Geometry check sheet. Reference: the model listing, model coordinates, mm. Face numbers are marked on the shaded views. A direction names the side the tool comes from. Round coordinates to 2 decimals unless told otherwise and drop trailing zeros. Order: outer loops, then holes, each group sorted by start corner. A loop starts at its lowest first (then second) coordinate and runs counter-clockwise, first axis right, second up.
(1) Sectioned sample at D-D (y = -21). Record the boundary of the cut face in (x, z).
(2) Sectioned sample at C-C (x = -4.5). Record the boundary of the cut face in (y, z), plus the area to 3 significant figures.
(3) Release check for a two-part mould opening along Z. For the marked faces 4, 5 and 6 record: +Z half, -Z half, draft (parallel to the pull), parting line (faces both ways), or undercut.
(4) Material ranges on line 1 along Y through (x, z) = (-3.75, -8); line 2 along Y through (x, z) = (6.25, -2); line 3 along Y through (x, z) = (2.25, -4), recorded low to high.
(5) Set-up check for the marked faces 1, 2 and 3: record each of +Z, -Z, +X, -X, +Y, -Y from which the full face is reachable in a straight line by a thin tool's end or side.
(6) Go/stop test with flat-tipped pins: pin 1 (2 mm diameter, centred on y = 9, z = 2, fed in from +X); pin 2 (1.5 mm diameter, centred on y = -34.5, z = 1, fed in from -X); pin 3 (4 mm diameter, centred on y = -15, z = -4.5, fed in from +X). Record where each tip stops, or that it passes through.
(7) Sectioned sample at A-A (y = -37). Record the boundary of the cut face in (x, z).
from build123d import *

# Parameters (mm, degrees)
CBORE_FOR_M3_SHCS1_D           = 3.4
CBORE_FOR_M3_SHCS1_DEPTH       = 8.5
CBORE_FOR_M3_SHCS1_CBORE_D     = 6.5
CBORE_FOR_M3_SHCS1_CBORE_DEPTH = 3
M3X0_5_TAPPED_HOLE1_D          = 2.5
CUT_EXTRUDE1_DEPTH             = 47.216880128
CUT_EXTRUDE1_DEPTH_BACK        = 47.216880128
SKETCH10_W                     = 1
SKETCH10_H                     = 15
CUT_EXTRUDE2_DEPTH             = 10


with BuildPart() as part:
    # Sketch1 → Revolve1 (revolve)
    with BuildSketch(Plane.XY):
        Polygon((-8.5, -44), (-8.5, -15.8), (-9.5, -15.8), (-9.5, -14), (-8.5, -14), (-8.5, 0), (-10, 0), (-10, 1.5), (-8.5, 1.5), (-8.5, 13.5), (-10, 13.5), (-10, 15), (0, 15), (0, -30), (-4, -30), (-4, -44), align=None)
    revolve(axis=Axis((0, 15, 0), (0, -1, 0)))

    # CBORE for M3 SHCS1
    with Locations(Plane.XY.offset(8.5)):
        with Locations((6.25, -37)):
            CounterBoreHole(CBORE_FOR_M3_SHCS1_D / 2, CBORE_FOR_M3_SHCS1_CBORE_D / 2, CBORE_FOR_M3_SHCS1_CBORE_DEPTH, depth=CBORE_FOR_M3_SHCS1_DEPTH)

    # M3x0.5 Tapped Hole1 (through all)
    with Locations(Plane.XY):
        with Locations((6.25, -37)):
            Hole(M3X0_5_TAPPED_HOLE1_D / 2)

    # Sketch10 → Cut-Extrude1 (cut, two sides: drawn at the far end of the back side and taken through both)
    with BuildSketch(Plane(origin=(0, 0, 0), x_dir=(0, 0, -1), z_dir=(1, 0, 0)).offset(-CUT_EXTRUDE1_DEPTH_BACK)):
        with Locations((0, -37.5)):
            Rectangle(SKETCH10_W, SKETCH10_H)
    extrude(amount=CUT_EXTRUDE1_DEPTH + CUT_EXTRUDE1_DEPTH_BACK, mode=Mode.SUBTRACT)

    # Sketch10<3> → Cut-Extrude2 (cut)
    with BuildSketch(Plane(origin=(0, 0, 0), x_dir=(0, 0, -1), z_dir=(1, 0, 0))):
        Polygon((-0.5, -30), (0.5, -30), (9.5, -30), (9.5, -29), (-9.5, -29), (-9.5, -30), align=None)
    extrude(amount=CUT_EXTRUDE2_DEPTH, mode=Mode.SUBTRACT)


solid = part.part
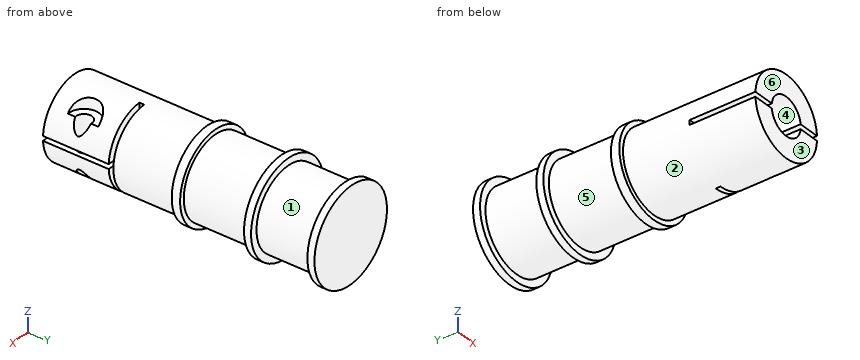
Answer below:
1. outline: circle Ø17 at (0, 0)
2. outline: (-44, -7.21) - (-15.8, -7.21) - (-15.8, -8.37) - (-14, -8.37) - (-14, -7.21) - (0, -7.21) - (0, -8.93) - (1.5, -8.93) - (1.5, -7.21) - (13.5, -7.21) - (13.5, -8.93) - (15, -8.93) - (15, 8.93) - (13.5, 8.93) - (13.5, 7.21) - (1.5, 7.21) - (1.5, 8.93) - (0, 8.93) - (0, 7.21) - (-14, 7.21) - (-14, 8.37) - (-15.8, 8.37) - (-15.8, 7.21) - (-44, 7.21) - (-44, 0.5) - (-30, 0.5) - (-30, -0.5) - (-44, -0.5) - close
2. area: 851 mm2
3. face 4: undercut
3. face 5: parting line
3. face 6: draft
4. line 1: y = -15.8 to -14, 0 to 1.5, 13.5 to 15
4. line 2: y = -44 to -38.25, -35.75 to -30, -29 to 15
4. line 3: y = -44 to -30, -29 to 15
5. face 1: none
5. face 2: -Y
5. face 3: +Z, -Z, +X, -X, -Y
6. pin 1: stops at x = 8.44
6. pin 2: stops at x = -8.49
6. pin 3: stops at x = 9.17
7. outline: (-8.49, -0.5) arc R8.5 ccw to (5, -6.87) - (5, -0.5) - (3.97, -0.5) arc R4 cw to (-3.97, -0.5) - close; (-8.49, 0.5) - (-3.97, 0.5) arc R4 cw to (3.97, 0.5) - (4.55, 0.5) - (4.55, 5.5) - (3, 5.5) - (3, 7.95) arc R8.5 ccw to start; (7.5, -4) arc R8.5 ccw to (8.49, -0.5) - (7.5, -0.5) - close; (7.95, 0.5) - (8.49, 0.5) arc R8.5 ccw to (7.95, 3.01) - close
